Verification items for the finished model (mm, model axes). A direction names the side the tool comes from. Round coordinates to 2 decimals unless told otherwise and drop trailing zeros. Order: outer loops, then holes, each group sorted by start corner. A loop starts at its lowest first (then second) coordinate and runs counter-clockwise, first axis right, second up.
```python
from build123d import *

# Parameters (mm, degrees)
F1_DEPTH = 68.072
F2_DEPTH = 25.4


with BuildPart() as f1:
    # F0 (on Front) → F1 (new body)
    with BuildSketch(Plane.XZ):
        Polygon((63.0641430616, 62.1895045042), (63.0641430616, 51.2399822474), (112.1140122414, 51.2399822474), (112.1140122414, 74.8909711838), (63.0641430616, 74.8909711838), align=None)
        Polygon((-49.4878217578, -17.0850455761), (49.4878217578, -17.0850455761), (49.4878217578, 17.0850455761), (-4.3794501107, 17.0850455761), (-49.4878217578, 17.0850455761), align=None)
        with BuildLine():
            Line((-4.3794501107, 17.0850455761), (49.4878217578, 17.0850455761))
            Line((49.4878217578, 17.0850455761), (49.4878217578, 38.5385379195))
            ThreePointArc((49.4878217578, 38.5385379195), (53.5207448585, 47.8342787205), (63.0641430616, 51.2399822474))
            Line((63.0641430616, 51.2399822474), (63.0641430616, 62.1895045042))
            Line((63.0641430616, 62.1895045042), (30.6561756879, 62.1895045042))
            ThreePointArc((30.6561756879, 62.1895045042), (6.4025600383, 56.5931809269), (-4.3794501107, 34.1587215662))
            Line((-4.3794501107, 34.1587215662), (-4.3794501107, 17.0850455761))
        make_face()
    extrude(amount=F1_DEPTH)

    # F2 (add): a face of the model
    f2_faces = [f1.faces().sort_by_distance(p)[0] for p in [
        (23.7821651341, -68.072, 24.4260783553),
    ]]
    extrude(f2_faces, amount=F2_DEPTH)


solid = f1.part
```
1) Sectioned sample at A-A on y = -37.5. Record the cut outline in (x, z), then the cut area to 3 significant figures.
2) Scan lines: probe 1 along Z at (x, y) = (35.5, -21); probe 2 along Z at (x, y) = (66.5, -17); probe 3 along X at (y, z) = (-7.5, 34). Record each from-to range of solid material in increasing order.
3) Tool access check on faces 1 (the flat face through (49.488, -46, 10)), 2 (the flat face through (30, 0, 30)), 3 (the flat face through (-27, -46, 17.085)). Record the directions out of +Z, -Z, +X, -X, +Y, -Y that give a thin tool (end or side, any length) a straight path to the whole face; none if there is none.
4) Sectioned sample at B-B on x = 47. Record the cut outline in (y, z).
5) Go/stop test with flat-tipped pins: pin 1 Ø10 at (y, z) = (-36, 10.5) entering from +X; pin 2 Ø1.5 at (y, z) = (-10.5, 27.5) entering from -X; pin 3 Ø3 at (x, y) = (-29, -51.5) entering from +Z. Record where each tip stops, or that it passes through.
6) Draft check along X on faces 4 (the flat face through (47, -46, 62.19)), 5 (the flat face through (-4.379, -46, 26)), 6 (the flat face through (-1, -46, -17.085)). Enter one of: released by +X, released by -X, zero draft, split by the parting line, or undercut.
7) Sectioned sample at C-C on z = 0.5. Record the cut outline in (x, y).
Returned:
1. outline: (-49.49, -17.09) - (49.49, -17.09) - (49.49, 38.54) arc R12.73 cw to (63.06, 51.24) - (112.11, 51.24) - (112.11, 74.89) - (63.06, 74.89) - (63.06, 62.19) - (30.66, 62.19) arc R28.73 ccw to (-4.38, 34.16) - (-4.38, 17.09) - (-49.49, 17.09) - close
1. area: 7,000 mm2
2. probe 1: z = -17.09 to 62.19
2. probe 2: z = 51.24 to 74.89
2. probe 3: x = -4.38 to 49.49
3. face 1: -Z, +X, +Y, -Y
3. face 2: +Z, -Z, +X, -X, +Y
3. face 3: +Z, -X, +Y, -Y
4. outline: (-93.47, -17.09) - (0, -17.09) - (0, 62.19) - (-93.47, 62.19) - close
5. pin 1: stops at x = 49.49
5. pin 2: stops at x = -4.38
5. pin 3: stops at z = 17.09
6. face 4: undercut
6. face 5: released by -X
6. face 6: zero draft
7. outline: (-49.49, -93.47) - (49.49, -93.47) - (49.49, 0) - (-49.49, 0) - close
